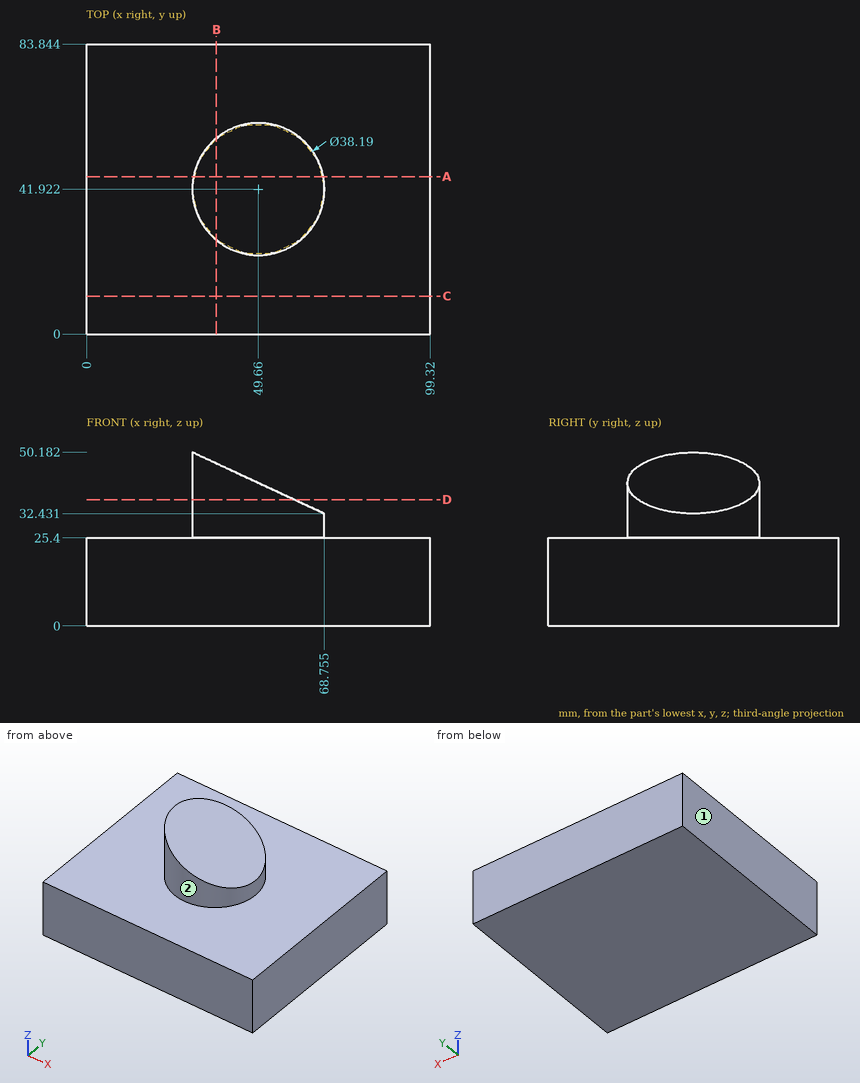
Here's the drawing with two shaded views (mm, measured from the low corner). I have some questions. A direction names the side the tool comes from. Round coordinates to 2 decimals unless told otherwise and drop trailing zeros. Order: outer loops, then holes, each group sorted by start corner. A loop starts at its lowest first (then second) coordinate and runs counter-clockwise, first axis right, second up. Notation, with made-up numbers: M 55.25,-13 L 66.25,-13 A35 ccw 66.25,24 Z; hole C 19,41 d5. An arc over 180 degrees is marked long. Answer in a Markdown table with one row per item.
Item 1: Imagine slicing it at C-C, the plane y = 11. Write out the boundary of the cut face in (x, z).
A:
| item | result |
|---|---|
| outline | M 0,0 L 99.32,0 L 99.32,25.4 L 0,25.4 Z |
Item 2: Imagine slicing it at B-B, the plane x = 37.5. Write out the boundary of the cut face in (y, z) (1 decimal), and give its area (3 significant figures).
A:
| item | result |
|---|---|
| outline | M 0,0 L 83.8,0 L 83.8,25.4 L 56.6,25.4 L 56.6,47 L 27.2,47 L 27.2,25.4 L 0,25.4 Z |
| area | 2,760 mm2 |
Item 3: For the marked faces 1 and 2, which set-ups out of +Z, -Z, +X, -X, +Y, -Y let a thin tool reach every point of the face, with its end or its side?
A:
| item | result |
|---|---|
| face 1 | +Z, -Z, -X, +Y, -Y |
| face 2 | +Z |
Item 4: If I drill on L1, parallel to Z at x = 40, y = 16; L2, parallel to Y at x = 32.5, z = 39 (1 decimal); L3, parallel to Z at x = 45, y = 47.5, over which ranges is the centre line in solid material (lowest first)? Write a range as from..to.
A:
| item | result |
|---|---|
| L1 | z = 0..25.4 |
| L2 | y = 33.5..50.3 |
| L3 | z = 0..43.47 |
Item 5: Imagine slicing it at D-D, the plane z = 36.5. Write out the boundary of the cut face in (x, y) (1 decimal), and give its area (3 significant figures).
A:
| item | result |
|---|---|
| outline | M 60,25.9 L 60,58 A19.1 ccw long Z |
| area | 947 mm2 |
Item 6: Imagine slicing it at A-A, the plane y = 45.5. Write out the boundary of the cut face in (x, z) (1 decimal), and give its area (3 significant figures).
A:
| item | result |
|---|---|
| outline | M 0,0 L 99.3,0 L 99.3,25.4 L 68.4,25.4 L 68.4,32.6 L 30.9,50 L 30.9,25.4 L 0,25.4 Z |
| area | 3,120 mm2 |
Item 7: I'm going to push flat-ended pins straight in: pin 1 (3 mm diameter, centred on x = 51, y = 28, fed in from +Z); pin 2 (1 mm diameter, centred on x = 60, z = 28.5, fed in from +Y); pin 3 (2 mm diameter, centred on x = 44.5, z = 30.5, fed in from +Y). Where does each tip first touch, or does it pass through?
A:
| item | result |
|---|---|
| pin 1 | stops at z = 41.38 |
| pin 2 | stops at y = 58.29 |
| pin 3 | stops at y = 60.56 |
